Autodesk Inventor part; units mm, degrees
ref_plane "ANBAU_XY" through (0, 0, 0) normal (0, 0, -1) x (1, 0, 0)
ref_plane "ANBAU_YZ" through (0, 0, 0) normal (1, 0, 0) x (0, -1, 0)
ref_plane "ANBAU_ZX" through (0, 0, 0) normal (0, -1, 0) x (0, 0, -1)
sketch "Sketch_1" plane through (0, 0, 0) normal (0, 0, 1) x (1, 0, 0)
  line L0 (-8.0829, 0) -> (-4.0415, -7)
  line L1 (-4.0415, -7) -> (4.0415, -7)
  line L2 (4.0415, -7) -> (8.0829, 0)
  line L3 (8.0829, 0) -> (4.0415, 7)
  line L4 (4.0415, 7) -> (-4.0415, 7)
  line L5 (-4.0415, 7) -> (-8.0829, 0)
extrude "Extrusion1" add sketch "Sketch_1" along normal blind 4
sketch "Sketch_2" plane through (0, 0, 0) normal (1, 0, 0) x (0, 1, 0)
  line L0 (0, 0) -> (0, 4)
  line L1 (0, 4) -> (5, 4)
  line L2 (5, 4) -> (4.4585, 3.4585)
  line L3 (4.4585, 3.4585) -> (4.4585, 0.5415)
  line L4 (4.4585, 0.5415) -> (5, 0)
  line L5 (5, 0) -> (0, 0)
  line L6 (0, 0) -> (0, 4)
revolve "Revolution1" cut sketch "Sketch_2" angle 360 about axis through (0, 0, 0) along (0, 0, -1)
thread "Thread1"
sketch "Sketch_3" plane through (0, 0, 0) normal (1, 0, 0) x (0, 1, 0)
  line L0 (0, -50) -> (0, 50)
  line L1 (17, 4) -> (7, 4)
  line L2 (7, 4) -> (13, 2.3923)
  line L3 (13, 2.3923) -> (13, 1.6077)
  line L4 (13, 1.6077) -> (7, 0)
  line L5 (7, 0) -> (17, 0)
  line L6 (17, 0) -> (17, 4)
revolve "Revolution2" cut sketch "Sketch_3" angle 360 about axis through (0, 0, -50) along (0, 0, -1)
ref_plane "ANBAU_XY" through (0, 0, 0) normal (0, 0, -1) x (1, 0, 0)
ref_plane "ANBAU_YZ" through (0, 0, 0) normal (1, 0, 0) x (0, -1, 0)
ref_plane "ANBAU_ZX" through (0, 0, 0) normal (0, -1, 0) x (0, 0, -1)
properties part number "5362901 M10x1"
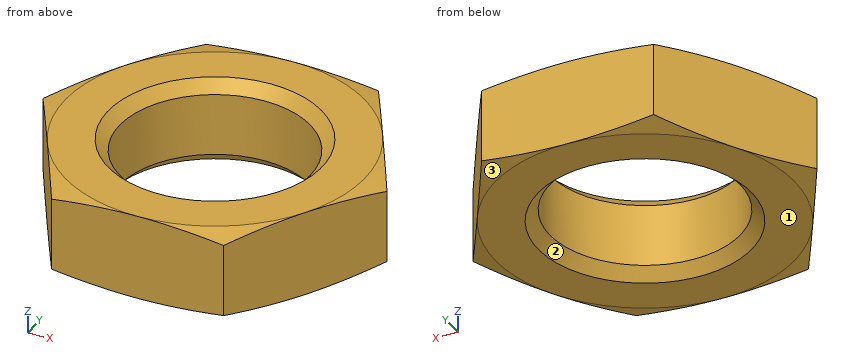
For this review, take the finished solid that the model builds, in its own axes (mm). Face numbers are marked on the shaded views. Round coordinates to 2 decimals unless told otherwise and drop trailing zeros. Loops run counter-clockwise (first coordinate to the right, second up) from the corner with the lowest first, then second, coordinate; pieces in that order, holes last.
(1) We need section A-A (z = 0.85). Give the boundary of the cut face in (x, y).
Returned:
outline: (-8.08, 0) - (-4.04, -7) - (4.04, -7) - (8.08, 0) - (4.04, 7) - (-4.04, 7) - close; hole circle Ø8.92 at (0, 0)
(2) Wall thickness on line 1 along Y through (x, z) = (-3, 2.35); line 2 along Y through (x, z) = (1.25, 2.8); line 3 along X through (y, z) = (-1.25, 1.25): over which ranges is each line inside the solid? List them lowest first.
Returned:
line 1: y = -7 to -3.3, 3.3 to 7
line 2: y = -7 to -4.28, 4.28 to 7
line 3: x = -7.36 to -4.28, 4.28 to 7.36
(3) Clearance check with a flat-ended pin moving along its axis: P1, Ø1, axis at x = 6, y = -4, coming from the +Z side. State where the tip first meets the part, or that it passes through.
Returned:
P1: stops at z = 4
(4) Mouldability with a two-part tool opening along X and no side actions: class the marked faces 1, 2 and 3 as released by +X, released by -X, zero draft, split by the parting line, or undercut.
Returned:
face 1: zero draft
face 2: undercut
face 3: released by +X
